Geometry check sheet. Reference: drawing and pictorial views, mm from the part's lowest x, y, z. Round coordinates to 2 decimals unless told otherwise and drop trailing zeros. Loops run counter-clockwise (first coordinate to the right, second up) from the corner with the lowest first, then second, coordinate; pieces in that order, holes last. Notation, with made-up numbers: M -8.5,12 L 5.5,12 A24 cw 5.5,30 Z; hole C 56.5,38.25 d6. An arc over 180 degrees is marked long. One line per question, with ' | ' between items. Start each with the question number.
(1) Section check B-B (z = 2.7). Count the separate pieces of the cut face and the enclosed holes in it, and give its area (3 significant figures).
(2) Section check C-C (y = 4.5). Record the boundary of the cut face in (x, z) (1 decimal).
(3) Section check A-A (x = 25). Record the boundary of the cut face in (y, z).
(4) Thickness scan on probe 1 along Y at (x, z) = (5, 1.55); probe 2 along X at (y, z) = (4.75, 2.2); probe 3 along X at (y, z) = (0.5, 0.7). Record the ranges inside material, lowest first. Write a range as [from, to].
(5) Section check D-D (y = 3). Record the boundary of the cut face in (x, z), and give its area (3 significant figures).
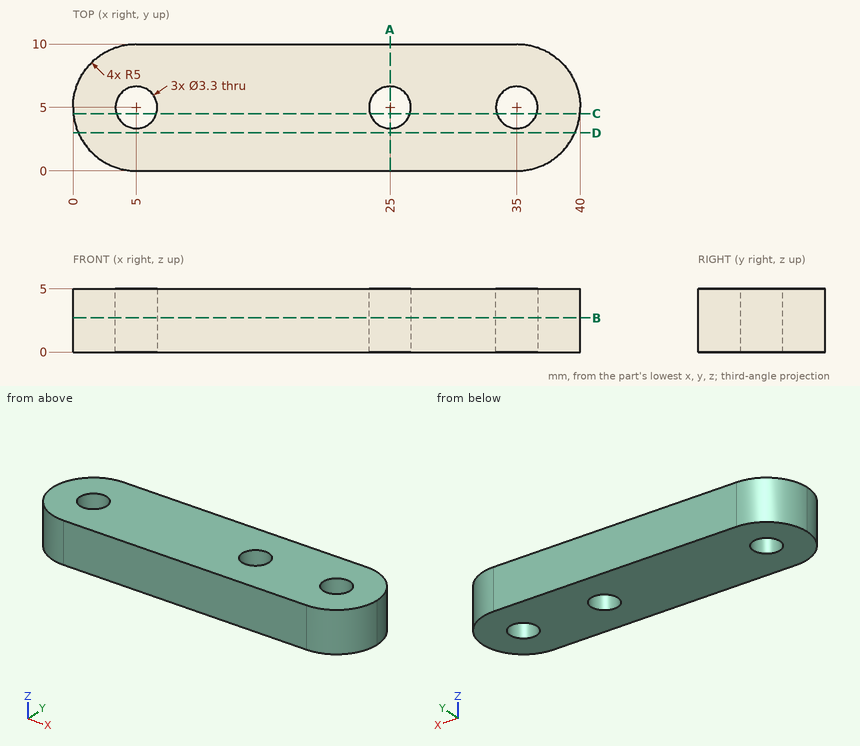
The answers:
1) separate pieces: 1 | enclosed holes: 3 | area: 353 mm²
2) outline: M 0,0 L 3.4,0 L 3.4,5 L 0,5 Z; M 6.6,0 L 23.4,0 L 23.4,5 L 6.6,5 Z; M 26.6,0 L 33.4,0 L 33.4,5 L 26.6,5 Z; M 36.6,0 L 40,0 L 40,5 L 36.6,5 Z
3) outline: M 0,0 L 3.35,0 L 3.35,5 L 0,5 Z; M 6.65,0 L 10,0 L 10,5 L 6.65,5 Z
4) probe 1: [0, 3.35], [6.65, 10] | probe 2: [0.01, 3.37], [6.63, 23.37], [26.63, 33.37], [36.63, 39.99] | probe 3: [2.82, 37.18]
5) outline: M 0.42,0 L 39.58,0 L 39.58,5 L 0.42,5 Z | area: 196 mm²
